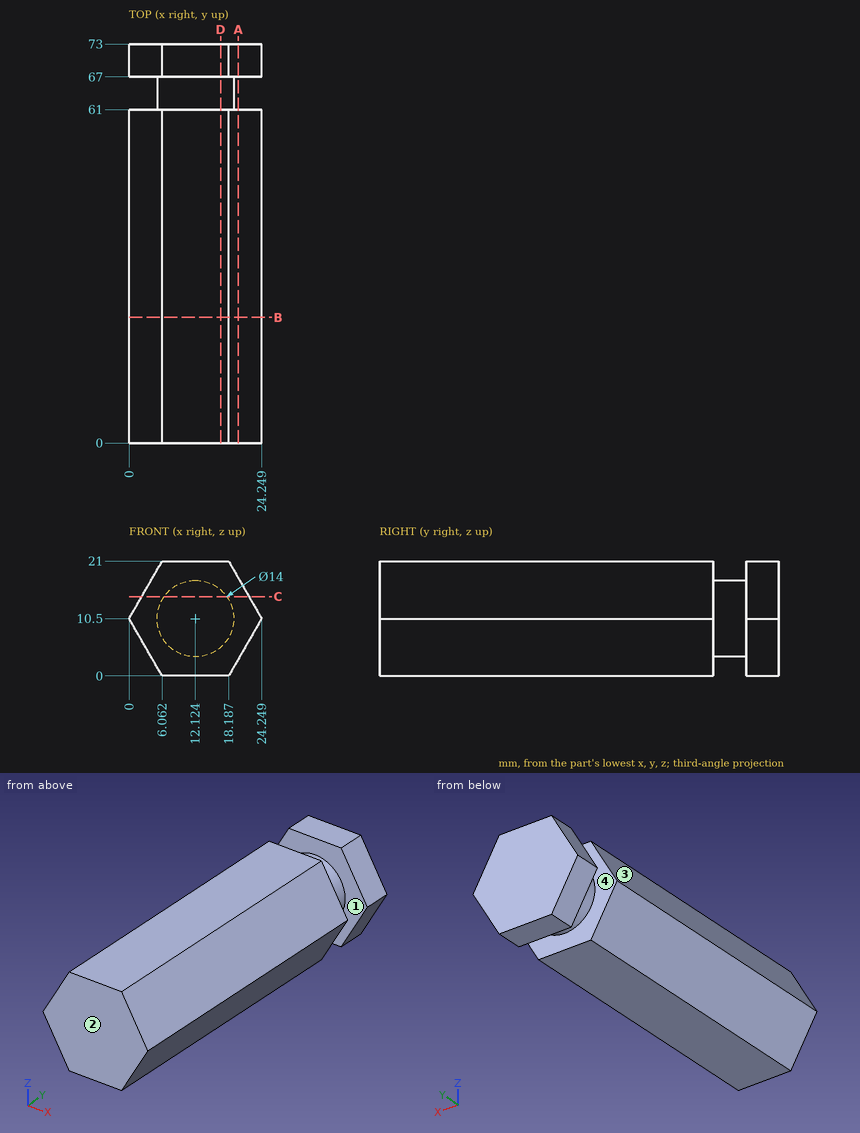
Answer from the drawing. Dimensions are ordinates in mm from the lowest x, y and z of the part. Give positions to 0.01 mm unless a question says otherwise; leave off trailing zeros. Write each loop counter-clockwise with the first axis right and the second up, starting at its lowest first coordinate (ties: lowest second). Pieces come first, ordered by that corner, then holes. Notation, with made-up numbers: (13.25, 24.5) - (17.25, 24.5) arc R18 cw to (17.25, 38.5) - close; hole circle Ø7 at (15.5, 48). An arc over 180 degrees is marked (long way). One line per item, written item: value. Start each with the question number.
1. Find section C-C (z = 14.5). Write down the section's boundary in (x, y).
2. Find section D-D (x = 16.75). Write down the section's boundary in (y, z), then the cut area to 3 significant figures.
3. Consider probe 1 along Y at (x, z) = (19.5, 7.5); probe 2 along X at (y, z) = (8.5, 16.5) (1 decimal); probe 3 along X at (y, z) = (64, 12.75) (1 decimal). Determine where each line is inside the solid, lowest interval first.
4. For a pull along Y with two mould halves and no side action, classify the marked faces 1, 2, 3 and 4 as +Y half, -Y half, draft (parallel to the pull), parting line (faces both ways), or undercut.
5. Given pin 1 (4 mm diameter, centred on y = 55, z = 4.5, fed in from -X); pin 2 (8 mm diameter, centred on y = 56.5, z = 15.5, fed in from -X); pin 3 (6 mm diameter, centred on x = 9.5, z = 16.5, fed in from -Y); pin 4 (2 mm diameter, centred on x = 3, z = 18, fed in from +Y), each flat-ended and moving along its own axis, determine where each tip first touches the part or whether it passes through.
6. Find section B-B (y = 23). Write down the section's boundary in (x, z).
7. Find section A-A (x = 20). Write down the section's boundary in (y, z), then the cut area to 3 significant figures.
Geometry results:
1. outline: (2.31, 0) - (21.94, 0) - (21.94, 61) - (17.87, 61) - (17.87, 67) - (21.94, 67) - (21.94, 73) - (2.31, 73) - (2.31, 67) - (6.38, 67) - (6.38, 61) - (2.31, 61) - close
2. outline: (0, 0) - (61, 0) - (61, 5.25) - (67, 5.25) - (67, 0) - (73, 0) - (73, 21) - (67, 21) - (67, 15.75) - (61, 15.75) - (61, 21) - (0, 21) - close
2. area: 1,470 mm2
3. probe 1: 0 to 61, 67 to 73
3. probe 2: 3.5 to 20.8
3. probe 3: 5.5 to 18.8
4. face 1: undercut
4. face 2: -Y half
4. face 3: draft
4. face 4: undercut
5. pin 1: x = 2.31
5. pin 2: x = 0.58
5. pin 3: y = 0
5. pin 4: through
6. outline: (0, 10.5) - (6.06, 0) - (18.19, 0) - (24.25, 10.5) - (18.19, 21) - (6.06, 21) - close
7. outline: (0, 3.14) - (61, 3.14) - (61, 17.86) - (0, 17.86) - close; (67, 3.14) - (73, 3.14) - (73, 17.86) - (67, 17.86) - close
7. area: 986 mm2
